Geometry check sheet. Reference: the model listing, model coordinates, mm. Face numbers are marked on the shaded views. Give positions to 0.01 mm unless a question says otherwise; leave off trailing zeros. Write each loop counter-clockwise with the first axis right and the second up, starting at its lowest first coordinate (ties: lowest second). Pieces come first, ordered by that corner, then holes. Notation, with made-up numbers: (44.25, 25) - (84.25, 25) arc R38 ccw to (84.25, 64) - close; hole circle Ø2 at (38, -12). An arc over 180 degrees is marked (long way). Use a Markdown table: item, result.
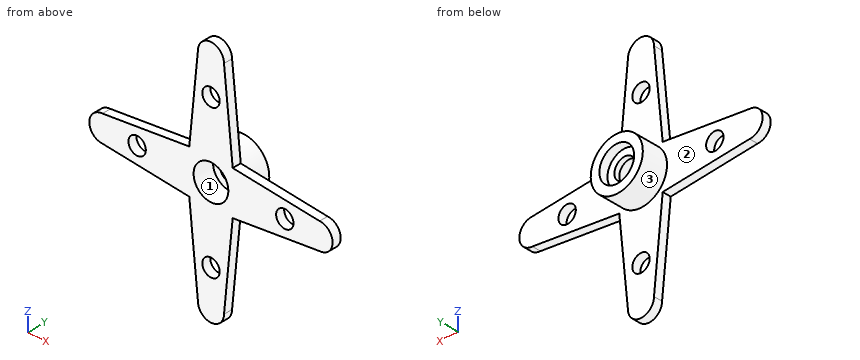
```python
from build123d import *

# Parameters (mm, degrees)
BOSS_EXTRUDE1_START     = -2.5
BOSS_EXTRUDE1_OUTLINE_R = 10
BOSS_EXTRUDE1_DEPTH     = 5
SKETCH2_R               = 15
SKETCH2_R_2             = 10
BOSS_EXTRUDE2_DEPTH     = 15
SKETCH3_R               = 5
CUT_EXTRUDE1_DEPTH      = 101.124921973
BOSS_EXTRUDE3_START     = 9.5
SKETCH4_R               = 10
SKETCH4_R_2             = 6
BOSS_EXTRUDE3_DEPTH     = 3


# Read off the part's stored shape, not the designer's step: Boss-Extrude1
with BuildPart() as part:
    # Boss-Extrude1 outline → Boss-Extrude1 (new body)
    with BuildSketch(Plane(origin=(0, 0, 0), x_dir=(1, 0, 0), z_dir=(0, 1, 0)).offset(BOSS_EXTRUDE1_START)):
        with BuildLine():
            Line((12.5, 12.5), (7.5, 62.5))
            ThreePointArc((7.5, 62.5), (0, 70), (-7.5, 62.5))
            Line((-7.5, 62.5), (-12.5, 12.5))
            Line((-12.5, 12.5), (-62.5, 7.5))
            ThreePointArc((-62.5, 7.5), (-70, 0), (-62.5, -7.5))
            Line((-62.5, -7.5), (-12.5, -12.5))
            Line((-12.5, -12.5), (-7.5, -62.5))
            ThreePointArc((-7.5, -62.5), (0, -70), (7.5, -62.5))
            Line((7.5, -62.5), (12.5, -12.5))
            Line((12.5, -12.5), (62.5, -7.5))
            ThreePointArc((62.5, -7.5), (70, 0), (62.5, 7.5))
            Line((62.5, 7.5), (12.5, 12.5))
        make_face()
        Circle(BOSS_EXTRUDE1_OUTLINE_R, mode=Mode.SUBTRACT)
    extrude(amount=BOSS_EXTRUDE1_DEPTH)

    # Sketch2 → Boss-Extrude2 (add)
    with BuildSketch(Plane(origin=(0, 2.5, 0), x_dir=(1, 0, 0), z_dir=(0, 1, 0))):
        with Locations(Location((0, 0, 0), (0, 0, 90))):
            Circle(SKETCH2_R)
        with Locations(Location((0, 0, 0), (0, 0, 270))):
            Circle(SKETCH2_R_2, mode=Mode.SUBTRACT)
    extrude(amount=BOSS_EXTRUDE2_DEPTH)

    # Sketch3 → Cut-Extrude1 (cut, through all)
    with BuildSketch(Plane(origin=(0, 2.5, 0), x_dir=(1, 0, 0), z_dir=(0, 1, 0))):
        with Locations(Location((42.5, 0, 0), (0, 0, 270))):
            Circle(SKETCH3_R)
        with Locations(Location((-42.5, 0, 0), (0, 0, 270))):
            Circle(SKETCH3_R)
        with Locations(Location((0, 42.5, 0), (0, 0, 270))):
            Circle(SKETCH3_R)
        with Locations(Location((0, -42.5, 0), (0, 0, 90))):
            Circle(SKETCH3_R)
    extrude(amount=-CUT_EXTRUDE1_DEPTH, mode=Mode.SUBTRACT)

    # Sketch4 → Boss-Extrude3 (add)
    with BuildSketch(Plane(origin=(0, 0, 0), x_dir=(1, 0, 0), z_dir=(0, 1, 0)).offset(BOSS_EXTRUDE3_START)):
        with Locations(Location((0, 0, 0), (0, 0, 270))):
            Circle(SKETCH4_R)
        with Locations(Location((0, 0, 0), (0, 0, 270))):
            Circle(SKETCH4_R_2, mode=Mode.SUBTRACT)
    extrude(amount=BOSS_EXTRUDE3_DEPTH)


solid = part.part
```
1) Depth check by flat-ended pin: P1, Ø11.5, axis at x = 0, z = 42.5, coming from the +Y side; P2, Ø19, axis at x = 0, z = 0, coming from the +Y side. Enter the tip coordinate at first touch or a pass-through.
Working result:
| item | result |
|---|---|
| P1 | stops at y = 2.5 |
| P2 | stops at y = 12.5 |
2) Material ranges on L1, parallel to X at y = 0.7, z = 0; L2, parallel to X at y = 3.25, z = 0; L3, parallel to Z at x = 6, y = 5, recorded low to high. Write a range as from..to.
Working result:
| item | result |
|---|---|
| L1 | x = -70..-47.5, -37.5..-10, 10..37.5, 47.5..70 |
| L2 | x = -15..-10, 10..15 |
| L3 | z = -13.75..-8, 8..13.75 |
3) Mould release check, pull along X, two halves, no side actions. Record for the marked faces 1, 2 and 3: pulls with the +X half, pulls with the -X half, needs draft (parallel to the pull), parting line crosses it, or undercut.
Working result:
| item | result |
|---|---|
| face 1 | undercut |
| face 2 | needs draft |
| face 3 | parting line crosses it |
4) Section check D-D on y = 6.5. Record the boundary of the cut face in (x, z), then the cut area to 3 significant figures.
Working result:
| item | result |
|---|---|
| outline | circle Ø30 at (0, 0); hole circle Ø20 at (0, 0) |
| area | 393 mm² |
5) Section check C-C on z = 39.5. Record the boundary of the cut face in (x, y).
Working result:
| item | result |
|---|---|
| outline | (-9.8, -2.5) - (-4, -2.5) - (-4, 2.5) - (-9.8, 2.5) - close; (4, -2.5) - (9.8, -2.5) - (9.8, 2.5) - (4, 2.5) - close |
6) Section check B-B on x = 0. Record the boundary of the cut face in (y, z).
Working result:
| item | result |
|---|---|
| outline | (-2.5, -70) - (2.5, -70) - (2.5, -47.5) - (-2.5, -47.5) - close; (-2.5, -37.5) - (2.5, -37.5) - (2.5, -15) - (17.5, -15) - (17.5, -10) - (12.5, -10) - (12.5, -6) - (9.5, -6) - (9.5, -10) - (-2.5, -10) - close; (-2.5, 10) - (9.5, 10) - (9.5, 6) - (12.5, 6) - (12.5, 10) - (17.5, 10) - (17.5, 15) - (2.5, 15) - (2.5, 37.5) - (-2.5, 37.5) - close; (-2.5, 47.5) - (2.5, 47.5) - (2.5, 70) - (-2.5, 70) - close |
7) Section check A-A on z = 0. Record the boundary of the cut face in (x, y), then the cut area to 3 significant figures.
Working result:
| item | result |
|---|---|
| outline | (-70, -2.5) - (-47.5, -2.5) - (-47.5, 2.5) - (-70, 2.5) - close; (-37.5, -2.5) - (-10, -2.5) - (-10, 9.5) - (-6, 9.5) - (-6, 12.5) - (-10, 12.5) - (-10, 17.5) - (-15, 17.5) - (-15, 2.5) - (-37.5, 2.5) - close; (6, 9.5) - (10, 9.5) - (10, -2.5) - (37.5, -2.5) - (37.5, 2.5) - (15, 2.5) - (15, 17.5) - (10, 17.5) - (10, 12.5) - (6, 12.5) - close; (47.5, -2.5) - (70, -2.5) - (70, 2.5) - (47.5, 2.5) - close |
| area | 674 mm² |
